Source: CAD feature listing. Evaluate the final solid. Frame: model axes, mm. Face numbers are marked on the shaded views. A direction names the side the tool comes from. Give positions to 0.01 mm unless a question says otherwise; leave off trailing zeros. Order: outer loops, then holes, each group sorted by start corner. A loop starts at its lowest first (then second) coordinate and runs counter-clockwise, first axis right, second up.
from build123d import *

# Parameters (mm, degrees)
SKETCH1_W           = 5
SKETCH1_H           = 5
SKETCH1_W_2         = 3
SKETCH1_H_2         = 3
BOSS_EXTRUDE1_DEPTH = 6
BOSS_EXTRUDE2_REACH = 6
SKETCH2_W           = 3
SKETCH2_H           = 1
BOSS_EXTRUDE3_DEPTH = 1
SKETCH4_R           = 0.75
CUT_EXTRUDE2_DEPTH  = 1


with BuildPart() as part:
    # Sketch1 → Boss-Extrude1 (new body)
    with BuildSketch(Plane(origin=(0, 0, 0), x_dir=(1, 0, 0), z_dir=(0, 1, 0))):
        with Locations((2.5, 2.5)):
            Rectangle(SKETCH1_W, SKETCH1_H)
        with Locations((2.5, 2.5)):
            Rectangle(SKETCH1_W_2, SKETCH1_H_2, mode=Mode.SUBTRACT)
    extrude(amount=BOSS_EXTRUDE1_DEPTH)

    # Sketch2 → Boss-Extrude2 (add, up to next)
    with BuildSketch(Plane.XY.offset(-4), mode=Mode.PRIVATE) as boss_extrude2_sk1:
        with Locations((2.5, 5.5)):
            Rectangle(SKETCH2_W, SKETCH2_H)
    boss_extrude2_tool1 = extrude(boss_extrude2_sk1.sketch, amount=BOSS_EXTRUDE2_REACH, mode=Mode.PRIVATE) - part.part
    add(boss_extrude2_tool1.solids().sort_by_distance((2.5, 5.5, -4))[0])

    # Sketch3 → Boss-Extrude3 (add)
    with BuildSketch(Plane(origin=(0, 6, 0), x_dir=(1, 0, 0), z_dir=(0, 1, 0))):
        with BuildLine():
            ThreePointArc((3.560660172, 3.560660172), (2.5, 4), (1.439339828, 3.560660172))
            Line((1.439339828, 3.560660172), (2.5, 2.5))
            Line((2.5, 2.5), (3.560660172, 3.560660172))
        make_face()
        with BuildLine():
            Line((2.5, 2.5), (1.439339828, 3.560660172))
            ThreePointArc((1.439339828, 3.560660172), (1, 2.5), (1.439339828, 1.439339828))
            Line((1.439339828, 1.439339828), (2.5, 2.5))
        make_face()
        with BuildLine():
            Line((3.560660172, 3.560660172), (2.5, 2.5))
            Line((2.5, 2.5), (3.560660172, 1.439339828))
            ThreePointArc((3.560660172, 1.439339828), (3.885819299, 1.925974851), (4, 2.5))
            ThreePointArc((4, 2.5), (3.885819299, 3.074025149), (3.560660172, 3.560660172))
        make_face()
        with BuildLine():
            Line((3.560660172, 1.439339828), (2.5, 2.5))
            Line((2.5, 2.5), (1.439339828, 1.439339828))
            ThreePointArc((1.439339828, 1.439339828), (2.5, 1), (3.560660172, 1.439339828))
        make_face()
    extrude(amount=BOSS_EXTRUDE3_DEPTH)

    # Sketch4 → Cut-Extrude2 (cut)
    with BuildSketch(Plane.XZ.offset(-5)):
        with Locations((2.5, -2.5)):
            Circle(SKETCH4_R)
    extrude(amount=-CUT_EXTRUDE2_DEPTH, mode=Mode.SUBTRACT)


solid = part.part
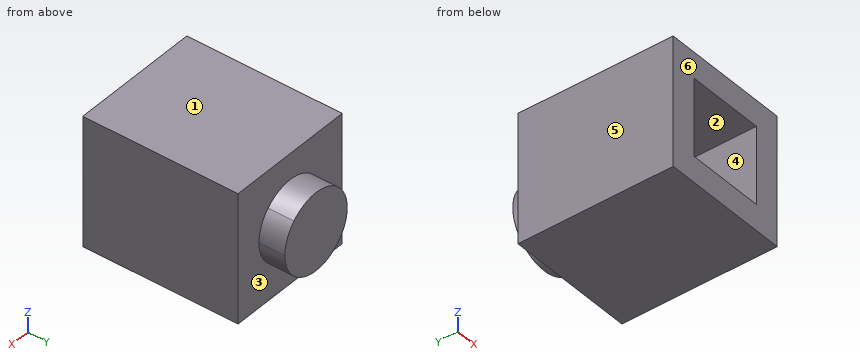
(1) Pin query (flat end, axial travel): pin 1 Ø1.5 at (x, z) = (2.5, -2) entering from -Y; pin 2 Ø1.2 at (x, z) = (2.5, -2.5) entering from -Y. Return the tip coordinate at first contact, or that it passes through.
(2) Section C-C, the plane z = -0.9. Return loops of the section in (x, y), plus the area to 3 significant figures.
(3) Line query: line 1 along Z through (x, y) = (2.5, 5.3); line 2 along Z through (x, y) = (2.35, 2); line 3 along X through (y, z) = (3.75, -3.65). Output: solid intervals per line, ascending.
(4) Section A-A, the plane y = 1.25. Return loops of the section in (x, z).
(5) Draft query along X for the marked faces 4, 5 and 6. Return one class per face: +X half, -X half, draft (parallel to the pull), parting line (faces both ways), or undercut.
(6) Section B-B, the plane x = 2.5. Return loops of the section in (y, z).
(7) Access query for the marked faces 1, 2 and 3. Directions: +Z, -Z, +X, -X, +Y, -Y. A direction counts if a zero-diameter tool reaches every point of the face in a straight line with its end or side. Return the directions, or none.
(8) Section D-D, the plane y = 5.25. Return loops of the section in (x, z).
Checks:
1. pin 1: stops at y = 5
1. pin 2: stops at y = 6
2. outline: (0, 0) - (5, 0) - (5, 6) - (0, 6) - close
2. area: 30.0 mm2
3. line 1: z = -5 to -3.25, -1.75 to 0
3. line 2: z = -5 to -4, -1 to 0
3. line 3: x = 0 to 1, 4 to 5
4. outline: (0, -5) - (5, -5) - (5, 0) - (0, 0) - close; hole (1, -4) - (4, -4) - (4, -1) - (1, -1) - close
5. face 4: undercut
5. face 5: -X half
5. face 6: draft
6. outline: (0, -5) - (6, -5) - (6, -4) - (7, -4) - (7, -1) - (6, -1) - (6, 0) - (0, 0) - (0, -1) - (5, -1) - (5, -1.75) - (6, -1.75) - (6, -3.25) - (5, -3.25) - (5, -4) - (0, -4) - close
7. face 1: +Z, +X, -X, +Y, -Y
7. face 2: -Y
7. face 3: +Y
8. outline: (0, -5) - (5, -5) - (5, 0) - (0, 0) - close; hole circle Ø1.5 at (2.5, -2.5)
